Source: CAD feature listing. Evaluate the final solid. Frame: model axes, mm. A direction names the side the tool comes from. Give positions to 0.01 mm unless a question says otherwise; leave off trailing zeros. Write each loop counter-clockwise with the first axis right and the second up, starting at its lowest first coordinate (ties: lowest second). Pieces come first, ordered by that corner, then holes. Notation, with made-up numbers: M -5.5,61 L 28.5,61 A34 cw 28.5,96 Z; hole C -11,-33.5 d2. An arc over 180 degrees is marked long. Return JSON: item names as keys, results as strings.
```python
from build123d import *

# Parameters (mm, degrees)
BOSS_EXTRUDE1_DEPTH = 50
SKETCH2_R           = 6
CUT_EXTRUDE1_DEPTH  = 12
FILLET1_R           = 12
FILLET2_R           = 12
RIB3_REACH          = 169.943
SKETCH14_WALL_W     = 393.768799168
SKETCH14_WALL_H     = 12
RIB5_REACH          = 169.943
SKETCH15_WALL_W     = 440.544630956
SKETCH15_WALL_H     = 12


with BuildPart() as part:
    # Sketch1 → Boss-Extrude1 (new, symmetric)
    with BuildSketch(Plane.XY):
        with BuildLine():
            Line((0, 0), (-12, 0))
            Line((-12, 0), (-12, 75))
            Line((-12, 75), (-24, 75))
            Line((-24, 75), (-24, 87))
            Line((-24, 87), (-12, 87))
            ThreePointArc((-12, 87), (-3.514718626, 83.485281374), (0, 75))
            Line((0, 75), (0, 40.485281374))
            Line((0, 40.485281374), (43.790729766, 84.27601114))
            ThreePointArc((43.790729766, 84.27601114), (41.248196059, 91.704696476), (41.476313815, 99.553123436))
            Line((41.476313815, 99.553123436), (21.28069991, 119.748737342))
            Line((21.28069991, 119.748737342), (29.765981284, 128.234018716))
            Line((29.765981284, 128.234018716), (55.928932188, 102.071067812))
            ThreePointArc((55.928932188, 102.071067812), (55.928932188, 87.928932188), (70.071067812, 87.928932188))
            Line((70.071067812, 87.928932188), (96.234018716, 61.765981284))
            Line((96.234018716, 61.765981284), (87.748737342, 53.28069991))
            Line((87.748737342, 53.28069991), (67.553123436, 73.476313815))
            ThreePointArc((67.553123436, 73.476313815), (59.704696476, 73.248196059), (52.27601114, 75.790729766))
            Line((52.27601114, 75.790729766), (0, 23.514718626))
            Line((0, 23.514718626), (0, 0))
        make_face()
    extrude(amount=BOSS_EXTRUDE1_DEPTH, both=True)

    # Sketch2 → Cut-Extrude1 (cut)
    with BuildSketch(Plane(origin=(79, 79, 0), x_dir=(0, 0, -1), z_dir=(0.7071067811865508, 0.7071067811865444, 0))):
        with Locations(Location((-38, 57.627416998, 0), (0, 0, 90))):
            Circle(SKETCH2_R)
        with Locations(Location((38, 57.627416998, 0), (0, 0, 90))):
            Circle(SKETCH2_R)
        with Locations(Location((38, -12.372583002, 0), (0, 0, 90))):
            Circle(SKETCH2_R)
        with Locations(Location((-38, -12.372583002, 0), (0, 0, 90))):
            Circle(SKETCH2_R)
    extrude(amount=-CUT_EXTRUDE1_DEPTH, mode=Mode.SUBTRACT)

    # Fillet1
    fillet1_edges = [part.edges().sort_by_distance(p)[0] for p in [
        (91.991378029, 57.523340597, 50),
        (25.523340597, 123.991378029, -50),
        (91.991378029, 57.523340597, -50),
        (25.523340597, 123.991378029, 50),
    ]]
    fillet(fillet1_edges, radius=FILLET1_R)

    # Fillet2
    fillet2_edges = [part.edges().sort_by_distance(p)[0] for p in [
        (-6, 0, -50),
        (-6, 0, 50),
    ]]
    fillet(fillet2_edges, radius=FILLET2_R)

    # Sketch14 wall → Rib3 (add, up to next)
    with BuildSketch(Plane(origin=(-1.359650045, 103.374368671, 0), x_dir=(-0.810288257242, -0.586031518074, 0), z_dir=(0.586031518074, -0.810288257242, 0)), mode=Mode.PRIVATE) as rib3_sk1:
        Rectangle(SKETCH14_WALL_W, SKETCH14_WALL_H)
    rib3_tool1 = extrude(rib3_sk1.sketch, amount=RIB3_REACH, mode=Mode.PRIVATE) - part.part
    add(rib3_tool1.solids().sort_by_distance((-1.359650045, 103.374368671, 0))[0])

    # Sketch15 wall → Rib5 (add, up to next)
    with BuildSketch(Plane(origin=(43.874368671, 26.640349955, 0), x_dir=(-0.854767287398, -0.519011449193, 0), z_dir=(0.519011449193, -0.854767287398, 0)), mode=Mode.PRIVATE) as rib5_sk1:
        Rectangle(SKETCH15_WALL_W, SKETCH15_WALL_H)
    rib5_tool1 = extrude(rib5_sk1.sketch, amount=-RIB5_REACH, mode=Mode.PRIVATE) - part.part
    add(rib5_tool1.solids().sort_by_distance((43.874368671, 26.640349955, 0))[0])


solid = part.part
```
1) Cut plane D-D, the plane x = 63. Return the cut outline in (y, z).
Numbers:
{"outline": "M 38.25,-6 L 73,-6 L 73,-50 L 85,-50 L 85,50 L 73,50 L 73,6 L 38.25,6 Z"}
2) Cut plane B-B, the plane y = 47.5. Return the cut outline in (x, z), then the cut area to 3 significant figures.
Numbers:
{"outline": "M -12,-50 L 0,-50 L 0,-6 L 7.01,-6 L 7.01,-50 L 23.99,-50 L 23.99,-6 L 78.23,-6 L 78.23,6 L 23.99,6 L 23.99,50 L 7.01,50 L 7.01,6 L 0,6 L 0,50 L -12,50 Z", "area": "3,630 mm²"}
3) Contact query for flat-ended pins moving along their axis: pin 1 Ø7 at (y, z) = (11.5, -27.5) entering from +X; pin 2 Ø10 at (x, y) = (45, 54) entering from +Z; pin 3 Ø1.5 at (y, z) = (107, 33.5) entering from -X; pin 4 Ø9.5 at (x, z) = (-15, 19) entering from -Y. Output: stop coordinate, or through.
Numbers:
{"pin 1": "stops at x = 0", "pin 2": "stops at z = 6", "pin 3": "stops at x = 33.28", "pin 4": "stops at y = 0"}
4) Draft query along X for faces 5 (the face through (26.504, 50.019, -27.692)), 6 (the face through (89.38, 60.02, -46.58)), 7 (the face through (59.814, 73.232, 28.308)), 8 (the face through (25.46, 123.93, 0.53)). Return one class per face: released by +X, released by -X, zero draft, split by the parting line, or undercut.
Numbers:
{"face 5": "undercut", "face 6": "released by +X", "face 7": "undercut", "face 8": "released by -X"}
5) Set-up query: faces 1 (the face through (-18, 87, -28)), 2 (the face through (13, 82, -6)), 3 (the face through (-18, 87, 28)), 4 (the face through (37, 39, -6)). Return all of +Z, -Z, +X, -X, +Y, -Y with unobstructed straight access to the full face (end or side cutting, diameter ignored); none if empty.
Numbers:
{"face 1": "-Z, -X, +Y", "face 2": "-Z", "face 3": "+Z, -X, +Y", "face 4": "-Z, -Y"}
6) Cut plane A-A, the plane z = -36. Return the cut outline in (x, y).
Numbers:
{"outline": "M -24,75 L -12,75 L -12,0 L 0,0 L 0,23.51 L 52.28,75.79 A22 ccw 67.55,73.48 L 75.26,65.77 L 83.75,74.25 L 70.07,87.93 A10 cw 55.93,102.07 L 42.25,115.75 L 33.77,107.26 L 41.48,99.55 A22 ccw 43.79,84.28 L 0,40.49 L 0,75 A12 ccw -12,87 L -24,87 Z; M 21.28,119.75 L 25.77,115.26 L 34.25,123.75 L 29.77,128.23 Z; M 83.26,57.77 L 87.75,53.28 L 96.23,61.77 L 91.75,66.25 Z"}
7) Line query: line 1 (X direction, y = 64, z = -26); line 2 (X direction, y = 29.5, z = -19); line 3 (Z direction, x = 61, y = 38.5). Output: solid intervals per line, ascending. Write a range as [from, to].
Numbers:
{"line 1": "x = [-12, 0], [23.51, 40.49], [77.03, 94]", "line 2": "x = [-12, 5.99]", "line 3": "z = [-6, 6]"}
8) Cut plane C-C, the plane z = -3.5. Return the cut outline in (x, y).
Numbers:
{"outline": "M -24,75 L -12,75 L -12,0 L 0,0 L 87.75,53.28 L 96.23,61.77 L 70.07,87.93 A10 cw 55.93,102.07 L 29.77,128.23 L 21.28,119.75 L -24,87 Z"}
